```python
from build123d import *

# Parameters (mm, degrees)
F0_W     = 40
F0_H     = 4
F1_DEPTH = 4
F2_W     = 2
F2_H     = 54
F2_W_2   = 7.5
F2_H_2   = 4
F3_DEPTH = 4


with BuildPart() as f1:
    # F0 (on Front) → F1 (new body)
    with BuildSketch(Plane.XZ):
        Polygon((-54, 0), (-4, 0), (-4, 20), (0, 20), (0, 40), (-4, 40), (-4, 117), (0, 117), (-32.5, 277), (-15, 277), (-15, 362), (-69.5, 362), (-69.5, 358), (-109.5, 358), (-109.5, 362), (-140.5, 362), (-140.5, 358), (-180.5, 358), (-180.5, 362), (-235, 362), (-235, 277), (-217.5, 277), (-250, 117), (-246, 117), (-246, 40), (-250, 40), (-250, 20), (-246, 20), (-246, 0), (-196, 0), (-196, 4), (-146, 4), (-146, 0), (-104, 0), (-104, 4), (-54, 4), align=None)
        with Locations((-160.5, 275)):
            Rectangle(F0_W, F0_H, mode=Mode.SUBTRACT)
        with Locations((-89.5, 275)):
            Rectangle(F0_W, F0_H, mode=Mode.SUBTRACT)
    extrude(amount=F1_DEPTH)

    # F2 (on Front) → F3 (cut)
    with BuildSketch(Plane.XZ):
        with Locations((-33.5, 318)):
            Rectangle(F2_W, F2_H)
        with Locations((-216.5, 318)):
            Rectangle(F2_W, F2_H)
        with BuildLine():
            ThreePointArc((-125, 287), (-123.5857864376, 287.5857864376), (-123, 289))
            ThreePointArc((-123, 289), (-123.5857864376, 290.4142135624), (-125, 291))
            Line((-125, 291), (-125, 287))
        make_face()
        with Locations((-121.25, 37)):
            Rectangle(F2_W_2, F2_H_2)
        with Locations((-128.75, 37)):
            Rectangle(F2_W_2, F2_H_2)
        with Locations((-121.25, 126)):
            Rectangle(F2_W_2, F2_H_2)
        with Locations((-128.75, 126)):
            Rectangle(F2_W_2, F2_H_2)
        with Locations((-121.25, 215)):
            Rectangle(F2_W_2, F2_H_2)
        with Locations((-128.75, 215)):
            Rectangle(F2_W_2, F2_H_2)
        with BuildLine():
            Line((-125, 287), (-125, 291))
            ThreePointArc((-125, 291), (-127, 289), (-125, 287))
        make_face()
    extrude(amount=F3_DEPTH, mode=Mode.SUBTRACT)


solid = f1.part
```
CAD build for the part. Positions are in the model's coordinates, mm. A direction names the side the tool comes from. Coordinates: 2 decimals unless noted, no trailing zeros. Order: outer loops, then holes, each group sorted by start corner. A loop starts at its lowest first (then second) coordinate and runs counter-clockwise, first axis right, second up. Notation, with made-up numbers: (13.25, 39) - (64.25, 39) arc R31 ccw to (64.25, 78) - close; hole circle Ø5 at (-32, 15.25). An arc over 180 degrees is marked (long way). Answer in a Markdown table with one row per item.
1. Slice it at D-D, the plane z = 171.5. List the corners of the cut face in (x, y), then the cut area to 3 significant figures.
Answer:
| item | result |
|---|---|
| outline | (-238.93, -4) - (-11.07, -4) - (-11.07, 0) - (-238.93, 0) - close |
| area | 911 mm² |
2. Slice it at A-A, the plane x = -152. List the corners of the cut face in (y, z).
Answer:
| item | result |
|---|---|
| outline | (-4, 4) - (0, 4) - (0, 273) - (-4, 273) - close; (-4, 277) - (0, 277) - (0, 358) - (-4, 358) - close |
3. Drill centre lines: L1, parallel to X at y = -1.25, z = 293; L2, parallel to Z at x = -125, y = -1.1; L3, parallel to Z at x = -129, y = -1.15. Where is each one in solid material? Low to high. Write a range as from..to.
Answer:
| item | result |
|---|---|
| L1 | -235..-217.5, -215.5..-34.5, -32.5..-15 |
| L2 | 0..35, 39..124, 128..213, 217..287, 291..362 |
| L3 | 0..35, 39..124, 128..213, 217..362 |
4. Slice it at B-B, the plane y = -2.2. Give the number of separate pieces and of enclosed holes in the cut face, then the cut area to 3 significant figures.
Answer:
| item | result |
|---|---|
| separate pieces | 1 |
| enclosed holes | 8 |
| area | 80,500 mm² |
5. Flat gauge pins, fed straight in: P1, Ø2, axis at y = -0.5, z = 205.5, coming from the -X side; P2, Ø2, axis at y = -2, z = 190, coming from the +X side (3 decimals); P3, Ø2, axis at y = -2.5, z = 215.5, coming from the +X side. Where does each tip first touch, or does it go through?
Answer:
| item | result |
|---|---|
| P1 | x = -232.23 |
| P2 | x = -14.625 |
| P3 | x = -19.8 |
6. Pull direction Z, two halves, no side cores. Call faces 1 (the face through (-127, -4, 184)), 2 (the face through (-16.023, -1.972, 195.88)): +Z half, -Z half, draft (parallel to the pull), parting line (faces both ways), or undercut.
Answer:
| item | result |
|---|---|
| face 1 | draft |
| face 2 | undercut |
7. 3-axis set-ups, long thin cutter, end or side, ignore diameter. For faces 3 (the face through (-233.522, -1.972, 198.12)), 4 (the face through (-127, 0, 184)): which of +Z, -Z, +X, -X, +Y, -Y reach the whole face in a straight line?
Answer:
| item | result |
|---|---|
| face 3 | -X, +Y, -Y |
| face 4 | +Z, -Z, +X, -X, +Y |
8. Slice it at C-C, the plane x = -21. List the corners of the cut face in (y, z).
Answer:
| item | result |
|---|---|
| outline | (-4, 0) - (0, 0) - (0, 220.38) - (-4, 220.38) - close; (-4, 277) - (0, 277) - (0, 362) - (-4, 362) - close |
